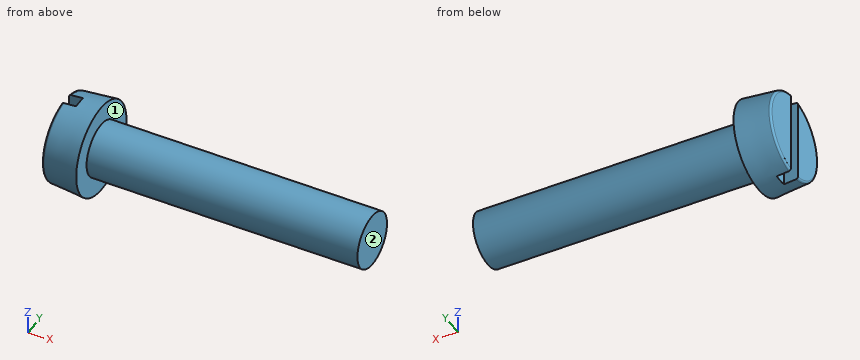
from build123d import *

# Parameters (mm, degrees)
FILLET2_R  = 0.2
SKETCH2_W  = 8.5
SKETCH2_H  = 1.2
SLOT_DEPTH = 1.3


with BuildPart() as part:
    # BodySke → Base-Revolve (revolve)
    with BuildSketch(Plane.XY):
        Polygon((3.3, 2.5), (3.3, 4.25), (0, 3.96128741), (0, 0), (28.3, 0), (28.3, 2.5), align=None)
    revolve(axis=Axis((-25.4, 0, 0), (1, 0, 0)))

    # Fillet2
    fillet2_edges = [part.edges().sort_by_distance(p)[0] for p in [
        (0, -3.96128741, 0),
    ]]
    fillet(fillet2_edges, radius=FILLET2_R)

    # Sketch2 → Slot (cut)
    with BuildSketch(Plane(origin=(0, 0, 0), x_dir=(0, 0, -1), z_dir=(1, 0, 0))):
        Rectangle(SKETCH2_W, SKETCH2_H)
    extrude(amount=SLOT_DEPTH, mode=Mode.SUBTRACT)


solid = part.part
Geometry check sheet. Reference: the model listing, model coordinates, mm. Face numbers are marked on the shaded views. A direction names the side the tool comes from. Coordinates: 2 decimals unless noted, no trailing zeros. Loops run counter-clockwise (first coordinate to the right, second up) from the corner with the lowest first, then second, coordinate; pieces in that order, holes last. Notation, with made-up numbers: (5, 83) - (27, 83) arc R23 cw to (27, 122) - close; hole circle Ø7 at (-7.5, -16). An arc over 180 degrees is marked (long way). Use one line per item in the form item = value. Start each with the question number.
Item 1: Section check A-A, the plane y = 0. Enter the section's corners in (x, z).
Item 2: Section check B-B, the plane x = 16.75. Enter the section's corners in (y, z), and give its area (3 significant figures).
Item 3: Thickness scan on probe 1 along X at (y, z) = (-3, 0.75); probe 2 along X at (y, z) = (0.25, -2.75); probe 3 along Z at (x, y) = (10.75, -1.25). Record the ranges inside material, lowest first.
Item 4: Tool access check on the marked faces 1 and 2. Record the directions out of +Z, -Z, +X, -X, +Y, -Y that give a thin tool (end or side, any length) a straight path to the whole face; none if there is none.
Item 5: Gauge pin test, flat ends, axial feed: pin 1 (5 mm diameter, centred on x = 15, z = 0.5, fed in from +Y); pin 2 (1 mm diameter, centred on x = 0.5, z = -1.5, fed in from -Y); pin 3 (1 mm diameter, centred on y = 0, z = -0.5, fed in from -X). Record the tip position at first contact, or that the pin passes through.
Computed:
q1.outline = (1.3, -4.08) - (3.3, -4.25) - (3.3, -2.5) - (28.3, -2.5) - (28.3, 2.5) - (3.3, 2.5) - (3.3, 4.25) - (1.3, 4.08) - close
q2.outline = circle Ø5 at (0, 0)
q2.area = 19.6 mm2
q3.probe_1 = 0 to 3.3
q3.probe_2 = 1.3 to 3.3
q3.probe_3 = -2.17 to 2.17
q4.face_1 = +X
q4.face_2 = +Z, -Z, +X, +Y, -Y
q5.pin_1 = 2.5
q5.pin_2 = -3.89
q5.pin_3 = 1.3
